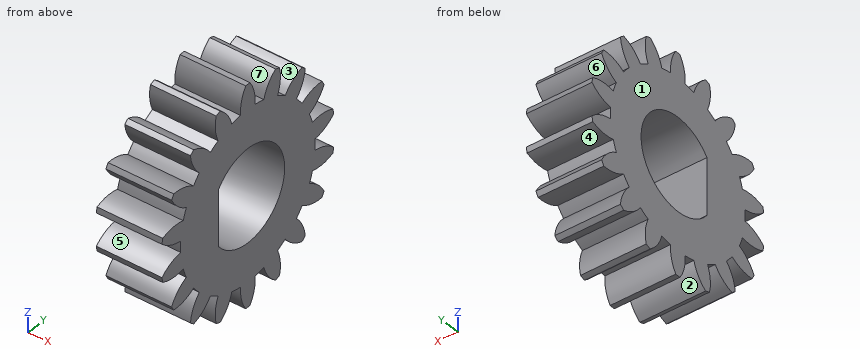
```python
from build123d import *

# Parameters (mm, degrees)
BASPROSKE_W        = 4
BASPROSKE_H        = 5
TOOTHCUT_DEPTH     = 9.124038405
TEETHCUTS_COUNT    = 18
TEETHCUTS_ANGLE    = 340
BORE_DEPTH         = 50.0000508
CUT_EXTRUDE1_DEPTH = 1


with BuildPart() as part:
    # BasProSke → Base-Revolve (revolve)
    with BuildSketch(Plane(origin=(0, 0, 0), x_dir=(1, 0, 0), z_dir=(0, 1, 0)), mode=Mode.PRIVATE) as base_revolve_sk:
        with Locations((2, 2.5)):
            Rectangle(BASPROSKE_W, BASPROSKE_H)
    revolve(base_revolve_sk.sketch.rotate(Axis((-10, 0, 0), (1, 0, 0)), 180), axis=Axis((-10, 0, 0), (1, 0, 0)))

    # TooCutSke → ToothCut (cut, through all)
    with BuildSketch(Plane(origin=(0, 0, 0), x_dir=(0, 0, -1), z_dir=(1, 0, 0))):
        with BuildLine():
            ThreePointArc((0.25527463, 3.865580275), (0, 3.874), (-0.25527463, 3.865580275))
            ThreePointArc((-0.25527463, 3.865580275), (-0.416281865, 4.46052923), (-0.768562654, 4.96628197))
            ThreePointArc((-0.768562654, 4.96628197), (0, 5.0254), (0.768562654, 4.96628197))
            ThreePointArc((0.768562654, 4.96628197), (0.416281865, 4.46052923), (0.25527463, 3.865580275))
        make_face()
    toothcut = extrude(amount=TOOTHCUT_DEPTH, mode=Mode.SUBTRACT)

    # TeethCuts: ToothCut ×18 about axis
    teethcuts_axis = Axis((-10, 0, 0), (1, 0, 0))
    for i in range(1, TEETHCUTS_COUNT):
        add(toothcut.rotate(teethcuts_axis, i * TEETHCUTS_ANGLE / (TEETHCUTS_COUNT - 1)), mode=Mode.SUBTRACT)

    # BorSke → Bore (cut, symmetric)
    with BuildSketch(Plane(origin=(0, 0, 0), x_dir=(0, 0, -1), z_dir=(1, 0, 0))):
        with BuildLine():
            Line((-1.295364774, -1.678222304), (1.295364774, -1.678222304))
            ThreePointArc((1.295364774, -1.678222304), (0, 2.12), (-1.295364774, -1.678222304))
        make_face()
    extrude(amount=BORE_DEPTH, both=True, mode=Mode.SUBTRACT)

    # Sketch1 → Cut-Extrude1 (cut)
    with BuildSketch(Plane.ZY):
        with BuildLine():
            ThreePointArc((3.220053404, 2.153864452), (3.645784857, 2.578031095), (3.908157867, 3.118701988))
            ThreePointArc((3.908157867, 3.118701988), (3.830222216, 3.213938048), (3.749966389, 3.30722725))
            ThreePointArc((3.749966389, 3.30722725), (3.171948906, 3.142726791), (2.680298817, 2.79711892))
            ThreePointArc((2.680298817, 2.79711892), (2.4901592, 2.967656173), (2.289195394, 3.125293658))
            ThreePointArc((2.289195394, 3.125293658), (2.544178562, 3.669488655), (2.605808207, 4.267289958))
            ThreePointArc((2.605808207, 4.267289958), (2.5, 4.330127019), (2.392677406, 4.390341084))
            ThreePointArc((2.392677406, 4.390341084), (1.905781113, 4.038067594), (1.561986006, 3.545148194))
            ThreePointArc((1.561986006, 3.545148194), (1.324986035, 3.640369213), (1.082226634, 3.719766325))
            ThreePointArc((1.082226634, 3.719766325), (1.135706785, 4.318351728), (0.98915962, 4.901179781))
            ThreePointArc((0.98915962, 4.901179781), (0.868240888, 4.924038765), (0.746796215, 4.943914988))
            ThreePointArc((0.746796215, 4.943914988), (0.409747992, 4.44635785), (0.25527463, 3.865580275))
            ThreePointArc((0.25527463, 3.865580275), (0, 3.874), (-0.25527463, 3.865580275))
            ThreePointArc((-0.25527463, 3.865580275), (-0.409747992, 4.44635785), (-0.746796215, 4.943914988))
            ThreePointArc((-0.746796215, 4.943914988), (-0.868240888, 4.924038765), (-0.98915962, 4.901179781))
            ThreePointArc((-0.98915962, 4.901179781), (-1.135706785, 4.318351728), (-1.082226634, 3.719766325))
            ThreePointArc((-1.082226634, 3.719766325), (-1.324986035, 3.640369213), (-1.561986006, 3.545148194))
            ThreePointArc((-1.561986006, 3.545148194), (-1.905781113, 4.038067594), (-2.392677406, 4.390341084))
            ThreePointArc((-2.392677406, 4.390341084), (-2.5, 4.330127019), (-2.605808207, 4.267289958))
            ThreePointArc((-2.605808207, 4.267289958), (-2.544178562, 3.669488655), (-2.289195394, 3.125293658))
            ThreePointArc((-2.289195394, 3.125293658), (-2.4901592, 2.967656173), (-2.680298817, 2.79711892))
            ThreePointArc((-2.680298817, 2.79711892), (-3.171948906, 3.142726791), (-3.749966389, 3.30722725))
            ThreePointArc((-3.749966389, 3.30722725), (-3.830222216, 3.213938048), (-3.908157867, 3.118701988))
            ThreePointArc((-3.908157867, 3.118701988), (-3.645784857, 2.578031095), (-3.220053404, 2.153864452))
            ThreePointArc((-3.220053404, 2.153864452), (-3.354982414, 1.937), (-3.475328033, 1.711715823))
            ThreePointArc((-3.475328033, 1.711715823), (-4.055532848, 1.868326755), (-4.654954082, 1.825213))
            ThreePointArc((-4.654954082, 1.825213), (-4.698463104, 1.710100717), (-4.739126009, 1.593952531))
            ThreePointArc((-4.739126009, 1.593952531), (-4.307655691, 1.175624937), (-3.762525451, 0.922647405))
            ThreePointArc((-3.762525451, 0.922647405), (-3.815145235, 0.67271304), (-3.851181399, 0.419854536))
            ThreePointArc((-3.851181399, 0.419854536), (-4.449959675, 0.368578939), (-4.998485613, 0.123051126))
            ThreePointArc((-4.998485613, 0.123051126), (-5, 0), (-4.998485613, -0.123051126))
            ThreePointArc((-4.998485613, -0.123051126), (-4.449959675, -0.368578939), (-3.851181399, -0.419854536))
            ThreePointArc((-3.851181399, -0.419854536), (-3.815145235, -0.67271304), (-3.762525451, -0.922647405))
            ThreePointArc((-3.762525451, -0.922647405), (-4.307655691, -1.175624937), (-4.739126009, -1.593952531))
            ThreePointArc((-4.739126009, -1.593952531), (-4.698463104, -1.710100717), (-4.654954082, -1.825213))
            ThreePointArc((-4.654954082, -1.825213), (-4.055532848, -1.868326755), (-3.475328033, -1.711715823))
            ThreePointArc((-3.475328033, -1.711715823), (-3.354982414, -1.937), (-3.220053404, -2.153864452))
            ThreePointArc((-3.220053404, -2.153864452), (-3.645784857, -2.578031095), (-3.908157867, -3.118701988))
            ThreePointArc((-3.908157867, -3.118701988), (-3.830222216, -3.213938048), (-3.749966389, -3.30722725))
            ThreePointArc((-3.749966389, -3.30722725), (-3.171948906, -3.142726791), (-2.680298817, -2.79711892))
            ThreePointArc((-2.680298817, -2.79711892), (-2.4901592, -2.967656173), (-2.289195394, -3.125293658))
            ThreePointArc((-2.289195394, -3.125293658), (-2.544178562, -3.669488655), (-2.605808207, -4.267289958))
            ThreePointArc((-2.605808207, -4.267289958), (-2.5, -4.330127019), (-2.392677406, -4.390341084))
            ThreePointArc((-2.392677406, -4.390341084), (-1.905781113, -4.038067594), (-1.561986006, -3.545148194))
            ThreePointArc((-1.561986006, -3.545148194), (-1.324986035, -3.640369213), (-1.082226634, -3.719766325))
            ThreePointArc((-1.082226634, -3.719766325), (-1.135706785, -4.318351728), (-0.98915962, -4.901179781))
            ThreePointArc((-0.98915962, -4.901179781), (-0.868240888, -4.924038765), (-0.746796215, -4.943914988))
            ThreePointArc((-0.746796215, -4.943914988), (-0.409747992, -4.44635785), (-0.25527463, -3.865580275))
            ThreePointArc((-0.25527463, -3.865580275), (0, -3.874), (0.25527463, -3.865580275))
            ThreePointArc((0.25527463, -3.865580275), (0.409747992, -4.44635785), (0.746796215, -4.943914988))
            ThreePointArc((0.746796215, -4.943914988), (0.868240888, -4.924038765), (0.98915962, -4.901179781))
            ThreePointArc((0.98915962, -4.901179781), (1.135706785, -4.318351728), (1.082226634, -3.719766325))
            ThreePointArc((1.082226634, -3.719766325), (1.324986035, -3.640369213), (1.561986006, -3.545148194))
            ThreePointArc((1.561986006, -3.545148194), (1.905781113, -4.038067594), (2.392677406, -4.390341084))
            ThreePointArc((2.392677406, -4.390341084), (2.5, -4.330127019), (2.605808207, -4.267289958))
            ThreePointArc((2.605808207, -4.267289958), (2.544178562, -3.669488655), (2.289195394, -3.125293658))
            ThreePointArc((2.289195394, -3.125293658), (2.4901592, -2.967656173), (2.680298817, -2.79711892))
            ThreePointArc((2.680298817, -2.79711892), (3.171948906, -3.142726791), (3.749966389, -3.30722725))
            ThreePointArc((3.749966389, -3.30722725), (3.830222216, -3.213938048), (3.908157867, -3.118701988))
            ThreePointArc((3.908157867, -3.118701988), (3.645784857, -2.578031095), (3.220053404, -2.153864452))
            ThreePointArc((3.220053404, -2.153864452), (3.354982414, -1.937), (3.475328033, -1.711715823))
            ThreePointArc((3.475328033, -1.711715823), (4.055532848, -1.868326755), (4.654954082, -1.825213))
            ThreePointArc((4.654954082, -1.825213), (4.698463104, -1.710100717), (4.739126009, -1.593952531))
            ThreePointArc((4.739126009, -1.593952531), (4.307655691, -1.175624937), (3.762525451, -0.922647405))
            ThreePointArc((3.762525451, -0.922647405), (3.815145235, -0.67271304), (3.851181399, -0.419854536))
            ThreePointArc((3.851181399, -0.419854536), (4.449959675, -0.368578939), (4.998485613, -0.123051126))
            ThreePointArc((4.998485613, -0.123051126), (5, 0), (4.998485613, 0.123051126))
            ThreePointArc((4.998485613, 0.123051126), (4.449959675, 0.368578939), (3.851181399, 0.419854536))
            ThreePointArc((3.851181399, 0.419854536), (3.815145235, 0.67271304), (3.762525451, 0.922647405))
            ThreePointArc((3.762525451, 0.922647405), (4.307655691, 1.175624937), (4.739126009, 1.593952531))
            ThreePointArc((4.739126009, 1.593952531), (4.698463104, 1.710100717), (4.654954082, 1.825213))
            ThreePointArc((4.654954082, 1.825213), (4.055532848, 1.868326755), (3.475328033, 1.711715823))
            ThreePointArc((3.475328033, 1.711715823), (3.354982414, 1.937), (3.220053404, 2.153864452))
        make_face()
    extrude(amount=-CUT_EXTRUDE1_DEPTH, mode=Mode.SUBTRACT)


solid = part.part
```
Here's how the part is built. I have some questions about the finished solid (model axes, mm). Face numbers are marked on the shaded views. A direction names the side the tool comes from. Coordinates: 2 decimals unless noted, no trailing zeros. Order: outer loops, then holes, each group sorted by start corner. A loop starts at its lowest first (then second) coordinate and runs counter-clockwise, first axis right, second up.
1) Which directions (+Z, -Z, +X, -X, +Y, -Y) give clear straight access to the entire face, cutting with the end or side of a thin tool? Please do the marked faces 5, 6 and 7.
2) We'd pull the mould along Z, two halves only. Please class the marked faces 1, 2, 3 and 4: +Z half, -Z half, draft (parallel to the pull), parting line (faces both ways), or undercut.
3) Imagine slicing it at B-B on y = 0. List the corners of the cut face in (x, z) for me, and give its area (3 significant figures).
4) Will these pins go through, and if not, where does the flat tip stop? pin 1 (1.5 mm diameter, centred on x = 2, y = 1.5, fed in from +Z); pin 2 (1.5 mm diameter, centred on x = 1.5, z = 3.5, fed in from -Y).
5) Imagine slicing it at A-A on z = 0. List the corners of the cut face in (x, y) for me.
6) I need wall thicknesses on line 1 (Y direction, x = 2.8, z = 0); line 2 (Y direction, x = 2.1, z = -4); line 3 (Z direction, x = 2.9, y = -4). Which ranges of each line are inside material? Lowest first, please.
7) Imagine slicing it at C-C on y = 4. List the corners of the cut face in (x, z) for me.
Response values:
1. face 5: +X, -X, -Y
1. face 6: +X, -X, +Y
1. face 7: +Z, +X, -X
2. face 1: draft
2. face 2: -Z half
2. face 3: +Z half
2. face 4: undercut
3. outline: (1, -5) - (4, -5) - (4, -2.12) - (1, -2.12) - close; (1, 2.12) - (4, 2.12) - (4, 5) - (1, 5) - close
3. area: 17.3 mm2
4. pin 1: stops at z = 4.74
4. pin 2: stops at y = -3.31
5. outline: (1, -3.87) - (4, -3.87) - (4, -1.68) - (1, -1.68) - close; (1, 2.12) - (4, 2.12) - (4, 3.87) - (1, 3.87) - close
6. line 1: y = -3.87 to -1.68, 2.12 to 3.87
6. line 2: y = -1.86 to -1.01, -0.43 to 0.43, 1.01 to 1.86
6. line 3: z = -2.6 to -1.87, -1.13 to -0.27, 0.27 to 1.13, 1.87 to 2.6
7. outline: (1, -2.6) - (4, -2.6) - (4, -1.87) - (1, -1.87) - close; (1, -1.13) - (4, -1.13) - (4, -0.27) - (1, -0.27) - close; (1, 0.27) - (4, 0.27) - (4, 1.13) - (1, 1.13) - close; (1, 1.87) - (4, 1.87) - (4, 2.6) - (1, 2.6) - close
